Source: CAD feature listing. Evaluate the final solid. Frame: model axes, mm. Round coordinates to 2 decimals unless told otherwise and drop trailing zeros. Write each loop counter-clockwise with the first axis right and the second up, starting at its lowest first coordinate (ties: lowest second). Pieces come first, ordered by that corner, then holes.
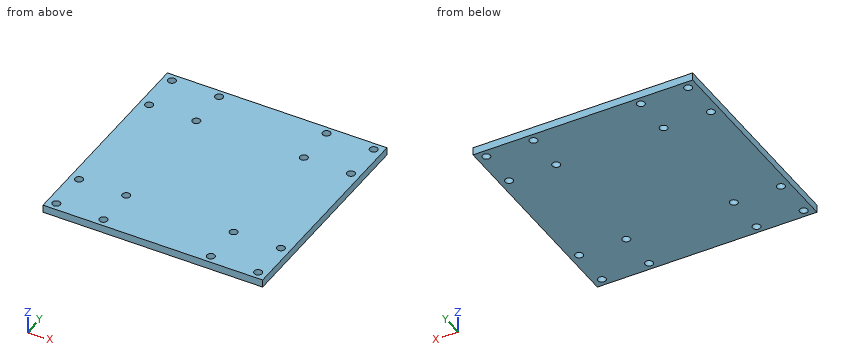
from build123d import *

# Parameters (mm, degrees)
SKETCH1_W           = 142
SKETCH1_H           = 142
BOSS_EXTRUDE1_DEPTH = 2.5
SKETCH2_R           = 2.55
CUT_EXTRUDE1_DEPTH  = 6


with BuildPart() as part:
    # Sketch1 → Boss-Extrude1 (new body, symmetric)
    with BuildSketch(Plane.XY):
        Rectangle(SKETCH1_W, SKETCH1_H)
    extrude(amount=BOSS_EXTRUDE1_DEPTH, both=True)

    # Sketch2 → Cut-Extrude1 (cut, through all)
    with BuildSketch(Plane.XY.offset(2.5)):
        with Locations((-65.25, 66)):
            Circle(SKETCH2_R)
        with Locations((-34.75, 66)):
            Circle(SKETCH2_R)
        with Locations((-34.75, 40)):
            Circle(SKETCH2_R)
        with Locations((-65.25, 40)):
            Circle(SKETCH2_R)
        with Locations((65.25, 66)):
            Circle(SKETCH2_R)
        with Locations((65.25, 40)):
            Circle(SKETCH2_R)
        with Locations((34.75, 40)):
            Circle(SKETCH2_R)
        with Locations((34.75, 66)):
            Circle(SKETCH2_R)
        with Locations((-65.25, -40)):
            Circle(SKETCH2_R)
        with Locations((-34.75, -40)):
            Circle(SKETCH2_R)
        with Locations((-34.75, -66)):
            Circle(SKETCH2_R)
        with Locations((-65.25, -66)):
            Circle(SKETCH2_R)
        with Locations((34.75, -40)):
            Circle(SKETCH2_R)
        with Locations((65.25, -40)):
            Circle(SKETCH2_R)
        with Locations((65.25, -66)):
            Circle(SKETCH2_R)
        with Locations((34.75, -66)):
            Circle(SKETCH2_R)
    extrude(amount=-CUT_EXTRUDE1_DEPTH, mode=Mode.SUBTRACT)


solid = part.part
1) Section query C-C on z = 1.65. State how many separate pieces and enclosed holes the cut face has, then the cut area to 3 significant figures.
Taken from the geometry:
separate pieces: 1
enclosed holes: 16
area: 19,800 mm2
2) Material intervals for line 1 (Y direction, x = -34.75, z = 1.1); line 2 (Y direction, x = -63, z = 0.5); line 3 (X direction, y = -64.5, z = 1.95), sorted ascending.
Taken from the geometry:
line 1: y = -71 to -68.55, -63.45 to -42.55, -37.45 to 37.45, 42.55 to 63.45, 68.55 to 71
line 2: y = -71 to -67.2, -64.8 to -41.2, -38.8 to 38.8, 41.2 to 64.8, 67.2 to 71
line 3: x = -71 to -67.31, -63.19 to -36.81, -32.69 to 32.69, 36.81 to 63.19, 67.31 to 71
3) Section query B-B on y = 66. Return the cut outline in (x, z), then the cut area to 3 significant figures.
Taken from the geometry:
outline: (-71, -2.5) - (-67.8, -2.5) - (-67.8, 2.5) - (-71, 2.5) - close; (-62.7, -2.5) - (-37.3, -2.5) - (-37.3, 2.5) - (-62.7, 2.5) - close; (-32.2, -2.5) - (32.2, -2.5) - (32.2, 2.5) - (-32.2, 2.5) - close; (37.3, -2.5) - (62.7, -2.5) - (62.7, 2.5) - (37.3, 2.5) - close; (67.8, -2.5) - (71, -2.5) - (71, 2.5) - (67.8, 2.5) - close
area: 608 mm2
4) Section query A-A on x = -34.75. Return the cut outline in (y, z), then the cut area to 3 significant figures.
Taken from the geometry:
outline: (-71, -2.5) - (-68.55, -2.5) - (-68.55, 2.5) - (-71, 2.5) - close; (-63.45, -2.5) - (-42.55, -2.5) - (-42.55, 2.5) - (-63.45, 2.5) - close; (-37.45, -2.5) - (37.45, -2.5) - (37.45, 2.5) - (-37.45, 2.5) - close; (42.55, -2.5) - (63.45, -2.5) - (63.45, 2.5) - (42.55, 2.5) - close; (68.55, -2.5) - (71, -2.5) - (71, 2.5) - (68.55, 2.5) - close
area: 608 mm2
5) Contact query for a flat-ended pin moving along its axis: P1, Ø6.5, axis at x = -65.25, y = -66, coming from the +Z side. Output: stop coordinate, or through.
Taken from the geometry:
P1: stops at z = 2.5
